```python
from build123d import *

# Parameters (mm, degrees)
SKETCH1_R           = 2.575
SKETCH1_R_2         = 1.575
BOSS_EXTRUDE1_DEPTH = 15
SKETCH2_R           = 3
SKETCH2_R_2         = 1.575
BOSS_EXTRUDE2_DEPTH = 3
CHAMFER1_SIZE       = 2.5
CHAMFER1_SIZE2      = 1


with BuildPart() as part:
    # Sketch1 → Boss-Extrude1 (new body)
    with BuildSketch(Plane(origin=(0, 0, 0), x_dir=(1, 0, 0), z_dir=(0, 1, 0))):
        Circle(SKETCH1_R)
        Circle(SKETCH1_R_2, mode=Mode.SUBTRACT)
    extrude(amount=BOSS_EXTRUDE1_DEPTH)

    # Sketch2 → Boss-Extrude2 (add)
    with BuildSketch(Plane(origin=(0, 15, 0), x_dir=(1, 0, 0), z_dir=(0, 1, 0))):
        Circle(SKETCH2_R)
        Circle(SKETCH2_R_2, mode=Mode.SUBTRACT)
    extrude(amount=-BOSS_EXTRUDE2_DEPTH)

    # Chamfer1
    chamfer1_edges = [part.edges().sort_by_distance(p)[0] for p in [
        (-3, 15, 0),
    ]]
    chamfer1_side = [part.faces().sort_by_distance(p)[0] for p in [
        (-3, 13.5, 0),
    ]]
    chamfer(chamfer1_edges, length=CHAMFER1_SIZE, length2=CHAMFER1_SIZE2, reference=chamfer1_side[0])


solid = part.part
```
Could you check a few things on this model? Use its own coordinates, in mm. A direction names the side the tool comes from. Give positions to 0.01 mm unless a question says otherwise; leave off trailing zeros. Loops run counter-clockwise (first coordinate to the right, second up) from the corner with the lowest first, then second, coordinate; pieces in that order, holes last. Notation, with made-up numbers: (85.25, -37) -> (139.25, -37) arc R20 cw to (139.25, -7) -> close; hole circle Ø7 at (-3, 30). An arc over 180 degrees is marked (long way). Put each result on its own line as item: value.
(1) For faces 1 (the face through (2.456, 5.916, -0.773)), 2 (the face through (-3, 12.3, -0.1)), which set-ups out of +Z, -Z, +X, -X, +Y, -Y let a thin tool reach every point of the face, with its end or its side?
Computed:
face 1: -Y
face 2: +Y, -Y
(2) Imagine slicing it at A-A on z = 0. Write out the boundary of the cut face in (x, y) (3 decimals), plus the area to 4 significant figures.
Computed:
outline: (-3, 12) -> (-2.575, 12) -> (-2.575, 0) -> (-1.575, 0) -> (-1.575, 15) -> (-2, 15) -> (-3, 12.5) -> close; (1.575, 0) -> (2.575, 0) -> (2.575, 12) -> (3, 12) -> (3, 12.5) -> (2, 15) -> (1.575, 15) -> close
area: 30.05 mm^2
(3) Thinking about a two-plate mould opening in Z: for faces 3 (the face through (0, 0, 2)), 4 (the face through (-0.28, 14.6, -2.14)), 5 (the face through (-1.25, 7.4, 0.96)), which applies, pulls with the +Z half, pulls with the -Z half, needs draft (parallel to the pull), parting line crosses it, or undercut?
Computed:
face 3: needs draft
face 4: parting line crosses it
face 5: undercut
(4) I'm going to push flat-ended pins straight in: pin 1 Ø2 at (x, y) = (1, 2) entering from +Z (3 decimals); pin 2 Ø3 at (x, z) = (0.5, 1.5) entering from -Y; pin 3 Ø1 at (y, z) = (2.5, -1) entering from +X; pin 4 Ø3 at (x, y) = (1, 7) entering from -Z (3 decimals). Where does each tip first touch, or does it pass through?
Computed:
pin 1: z = 2.575
pin 2: y = 0
pin 3: x = 2.53
pin 4: z = -2.575
(5) Please list where these lines run through material, in increasing order: probe 1 along X at (y, z) = (5, 0) (3 decimals); probe 2 along Z at (x, y) = (-0.9, 12.5). Write a range as [from, to].
Computed:
probe 1: [-2.575, -1.575], [1.575, 2.575]
probe 2: [-2.86, -1.29], [1.29, 2.86]
(6) Imagine slicing it at D-D on y = 13.25. Write out the boundary of the cut face in (x, z) (3 decimals).
Computed:
outline: circle Ø5.4 at (0, 0); hole circle Ø3.15 at (0, 0)
(7) Imagine slicing it at B-B on x = 0. Write out the boundary of the cut face in (y, z) (3 decimals).
Computed:
outline: (0, -2.575) -> (12, -2.575) -> (12, -3) -> (12.5, -3) -> (15, -2) -> (15, -1.575) -> (0, -1.575) -> close; (0, 1.575) -> (15, 1.575) -> (15, 2) -> (12.5, 3) -> (12, 3) -> (12, 2.575) -> (0, 2.575) -> close
(8) Imagine slicing it at C-C on y = 9.5. Write out the boundary of the cut face in (x, z) (3 decimals), plus the area to 3 significant figures.
Computed:
outline: circle Ø5.15 at (0, 0); hole circle Ø3.15 at (0, 0)
area: 13.0 mm^2
